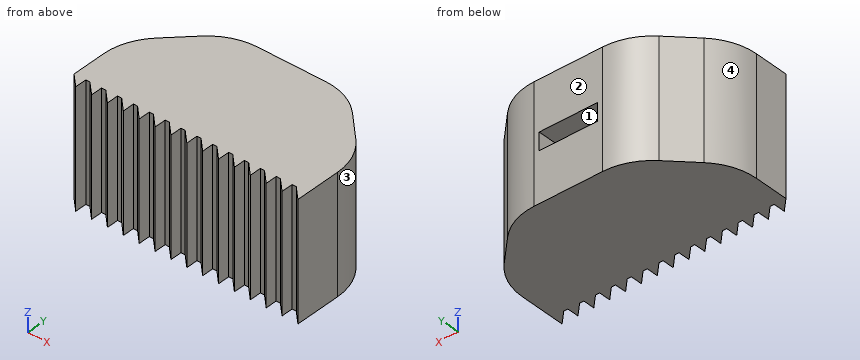
```python
from build123d import *

# Parameters (mm, degrees)
BOSS_EXTRUDE1_DEPTH = 20
SKETCH2_W           = 10
SKETCH2_H           = 3
CUT_EXTRUDE1_DEPTH  = 10
FILLET_1_R          = 10


with BuildPart() as part:
    # Sketch1 → Boss-Extrude1 (new body)
    with BuildSketch(Plane.XY):
        Polygon((17.014668726, -22), (17.014668726, -20), (17.728954441, -20), (19.728954441, -22), (19.728954441, -20), (19.728954441, -10), (9.728954441, 0), (-10.271045559, 0), (-20.271045559, -10), (-20.271045559, -20), (-18.271045559, -22), (-18.271045559, -20), (-17.556759845, -20), (-15.556759845, -22), (-15.556759845, -20), (-14.842474131, -20), (-12.842474131, -22), (-12.842474131, -20), (-12.128188417, -20), (-10.128188417, -22), (-10.128188417, -20), (-9.413902702, -20), (-7.413902702, -22), (-7.413902702, -20), (-6.699616988, -20), (-4.699616988, -22), (-4.699616988, -20), (-3.985331274, -20), (-1.985331274, -22), (-1.985331274, -20), (-1.271045559, -20), (0.728954441, -22), (0.728954441, -20), (1.443240155, -20), (3.443240155, -22), (3.443240155, -20), (4.157525869, -20), (6.157525869, -22), (6.157525869, -20), (6.871811583, -20), (8.871811583, -22), (8.871811583, -20), (9.586097298, -20), (11.586097298, -22), (11.586097298, -20), (12.300383012, -20), (14.300383012, -22), (14.300383012, -20), (15.014668726, -20), align=None)
    extrude(amount=BOSS_EXTRUDE1_DEPTH)

    # Sketch2 → Cut-Extrude1 (cut)
    with BuildSketch(Plane(origin=(0, 0, 0), x_dir=(1, 0, 0), z_dir=(0, 1, 0))):
        with Locations((-0.271045559, -10)):
            Rectangle(SKETCH2_W, SKETCH2_H)
    extrude(amount=-CUT_EXTRUDE1_DEPTH, mode=Mode.SUBTRACT)

    # Скругление1
    fillet_1_edges = [part.edges().sort_by_distance(p)[0] for p in [
        (-20.271045559, -10, 10),
        (-10.271045559, 0, 10),
        (9.728954441, 0, 10),
        (19.728954441, -10, 10),
    ]]
    fillet(fillet_1_edges, radius=FILLET_1_R)


solid = part.part
```
Read the model definition and answer for the solid it produces. Units are mm, in the model's axes. Face numbers are marked on the shaded views. Give positions to 0.01 mm unless a question says otherwise; leave off trailing zeros. Write each loop counter-clockwise with the first axis right and the second up, starting at its lowest first coordinate (ties: lowest second). Pieces come first, ordered by that corner, then holes. Notation, with made-up numbers: M 7,-13 L 66,-13 A17 ccw 66,19 Z; hole C -33,58.5 d3. An arc over 180 degrees is marked long. Put each result on its own line as item: value. Start each with the question number.
1. The part is cut by section A-A, the plane y = -8.75. Give the vertices of the cut face in (x, z).
2. Each of these flat-tipped pins is pushed along its axis until it touches: pin 1 Ø1 at (x, z) = (-10, 5.5) entering from -Y; pin 2 Ø0.8 at (x, z) = (-15, 12.5) entering from -Y; pin 3 Ø1.5 at (x, z) = (-14, 3) entering from +Y. Where does it stop, or does it pass through?
3. The part is cut by section B-B, the plane x = -3. Give the vertices of the cut face in (y, z), and give its area (3 significant figures).
4. Consider line 1 along Y through (x, z) = (-1, 14.75); line 2 along X through (y, z) = (-2, 15.5); line 3 along X through (y, z) = (-9, 15.75). Determine where each line is inside the solid, lowest interval first.
5. For a pull along X with two mould halves and no side action, classify the marked faces 1, 2, 3 and 4 as released by +X, released by -X, zero draft, split by the parting line, or undercut.
6. The part is cut by section D-D, the plane x = -11. Give the vertices of the cut face in (y, z), and give its area (3 significant figures).
7. The part is cut by section C-C, the plane y = -11.5. Give the vertices of the cut face in (x, z), and give its area (3 significant figures).
Final values:
1. outline: M -18.69,0 L 18.15,0 L 18.15,20 L -18.69,20 Z; hole M -5.27,8.5 L 4.73,8.5 L 4.73,11.5 L -5.27,11.5 Z
2. pin 1: stops at y = -22
2. pin 2: stops at y = -20.24
2. pin 3: stops at y = -2.98
3. outline: M -20.99,0 L 0,0 L 0,8.5 L -10,8.5 L -10,11.5 L 0,11.5 L 0,20 L -20.99,20 Z
3. area: 390 mm²
4. line 1: y = -20.27 to 0
4. line 2: x = -12.13 to 11.59
4. line 3: x = -18.85 to 18.31
5. face 1: undercut
5. face 2: zero draft
5. face 3: released by +X
5. face 4: released by -X
6. outline: M -21.13,0 L -1.27,0 L -1.27,20 L -21.13,20 Z
6. area: 397 mm²
7. outline: M -19.92,0 L 19.37,0 L 19.37,20 L -19.92,20 Z
7. area: 786 mm²
